Build history of the part. All positions in model axes, mm. A direction names the side the tool comes from. Coordinates: 2 decimals unless noted, no trailing zeros. Write each loop counter-clockwise with the first axis right and the second up, starting at its lowest first coordinate (ties: lowest second). Pieces come first, ordered by that corner, then holes. Notation, with made-up numbers: M -13,12 L 13,12 A26 ccw 13,38 Z; hole C -15,75 d4. An arc over 180 degrees is marked long. Use CSV: the item, a comma, the result in double quotes. Start each with the question number.
```python
from build123d import *

# Parameters (mm, degrees)
SKETCH1_R               = 3.75
BOSS_EXTRUDE1_DEPTH     = 5
CUT_EXTRUDE2_DEPTH      = 2
SKETCH4_R               = 3.75
SKETCH4_R_2             = 2.75
BOSS_EXTRUDE2_DEPTH     = 0.5
SKETCH5_W               = 2
SKETCH5_H               = 5
BOSS_EXTRUDE3_DEPTH     = 2
SKETCH5_2_W             = 2
SKETCH5_2_H             = 5
BOSS_EXTRUDE4_DEPTH     = 12
CUT_EXTRUDE3_DEPTH      = 121.241423811
CUT_EXTRUDE3_DEPTH_BACK = 121.241423811
SKETCH6_R               = 0.75
BOSS_EXTRUDE5_DEPTH     = 5


with BuildPart() as part:
    # Sketch1 → Boss-Extrude1 (new body)
    with BuildSketch(Plane.XY):
        with BuildLine():
            Line((120, 5), (120, -5))
            Line((120, -5), (0, -5))
            ThreePointArc((0, -5), (-5, 0), (0, 5))
            Line((0, 5), (120, 5))
        make_face()
        Circle(SKETCH1_R, mode=Mode.SUBTRACT)
    extrude(amount=BOSS_EXTRUDE1_DEPTH)

    # Sketch3 → Cut-Extrude2 (cut)
    with BuildSketch(Plane(origin=(0, 0, 0), x_dir=(-1, 0, 0), z_dir=(0, 0, -1))):
        with BuildLine():
            Line((-16.129718884, 2.749435925), (0, 4.1))
            ThreePointArc((0, 4.1), (4.1, 0), (0, -4.1))
            Line((0, -4.1), (-16.129718884, -2.749435925))
            ThreePointArc((-16.129718884, -2.749435925), (-18.4, 0), (-16.129718884, 2.749435925))
        make_face()
    extrude(amount=-CUT_EXTRUDE2_DEPTH, mode=Mode.SUBTRACT)

    # Sketch4 → Boss-Extrude2 (add)
    with BuildSketch(Plane(origin=(0, 0, 2), x_dir=(-1, 0, 0), z_dir=(0, 0, -1))):
        Circle(SKETCH4_R)
        Circle(SKETCH4_R_2, mode=Mode.SUBTRACT)
    extrude(amount=-BOSS_EXTRUDE2_DEPTH)

    # Sketch5 → Boss-Extrude3 (add)
    with BuildSketch(Plane(origin=(0, 5, 0), x_dir=(1, 0, 0), z_dir=(0, 1, 0))):
        with Locations((104, -2.5)):
            Rectangle(SKETCH5_W, SKETCH5_H)
    extrude(amount=BOSS_EXTRUDE3_DEPTH)

    # Sketch5<2> → Boss-Extrude4 (add)
    with BuildSketch(Plane(origin=(0, 5, 0), x_dir=(1, 0, 0), z_dir=(0, 1, 0))):
        with Locations((104, -2.5)):
            Rectangle(SKETCH5_2_W, SKETCH5_2_H)
    extrude(amount=-BOSS_EXTRUDE4_DEPTH)

    # Sketch6 → Cut-Extrude3 (cut, two sides: drawn at the far end of the back side and taken through both)
    with BuildSketch(Plane(origin=(0, 0, 2), x_dir=(-1, 0, 0), z_dir=(0, 0, -1)).offset(-CUT_EXTRUDE3_DEPTH_BACK)):
        with Locations((-17.55, 0)):
            Circle(SKETCH6_R)
        with BuildLine():
            ThreePointArc((-15.9, 0), (-15.15, -0.75), (-14.4, 0))
            Line((-14.4, 0), (-15.9, 0))
        make_face()
        with BuildLine():
            Line((-15.9, 0), (-14.4, 0))
            ThreePointArc((-14.4, 0), (-15.15, 0.75), (-15.9, 0))
        make_face()
        with BuildLine():
            ThreePointArc((-13.5, 0), (-12.75, -0.75), (-12, 0))
            Line((-12, 0), (-13.5, 0))
        make_face()
        with BuildLine():
            Line((-13.5, 0), (-12, 0))
            ThreePointArc((-12, 0), (-12.75, 0.75), (-13.5, 0))
        make_face()
        with BuildLine():
            ThreePointArc((-11.1, 0), (-10.35, -0.75), (-9.6, 0))
            Line((-9.6, 0), (-11.1, 0))
        make_face()
        with BuildLine():
            Line((-11.1, 0), (-9.6, 0))
            ThreePointArc((-9.6, 0), (-10.35, 0.75), (-11.1, 0))
        make_face()
        with BuildLine():
            ThreePointArc((-8.7, 0), (-7.95, -0.75), (-7.2, 0))
            Line((-7.2, 0), (-8.7, 0))
        make_face()
        with BuildLine():
            Line((-8.7, 0), (-7.2, 0))
            ThreePointArc((-7.2, 0), (-7.95, 0.75), (-8.7, 0))
        make_face()
    extrude(amount=CUT_EXTRUDE3_DEPTH + CUT_EXTRUDE3_DEPTH_BACK, mode=Mode.SUBTRACT)

    # Sketch7 → Boss-Extrude5 (add)
    with BuildSketch(Plane.XY.offset(5)):
        Polygon((120, 5), (127.743232655, 0), (120, -5), align=None)
    extrude(amount=-BOSS_EXTRUDE5_DEPTH)


solid = part.part
```
1. Slice it at B-B (x = 22.5). List the corners of the cut face in (y, z).
2. Drill centre lines: line 1 along Y through (x, z) = (7.95, 4.25); line 2 along Y through (x, z) = (0, 2.3); line 3 along Y through (x, z) = (28.5, 0.85). Where is each one in solid material? Low to high. Write a range as from..to.
3. 3-axis set-ups, long thin cutter, end or side, ignore diameter. For faces 1 (the flat face through (51, 5, 2)), 2 (the flat face through (7, -1, 2)), 3 (the cylindrical face through (-3.746, 0.165, 3.732)), 4 (the flat face through (113, -5, 2)), 5 (the flat face through (52, -5, 2)): which of +Z, -Z, +X, -X, +Y, -Y reach the whole face in a straight line?
4. Flat gauge pins, fed straight in: pin 1 (8 mm diameter, centred on x = -2, y = 1, fed in from +Z); pin 2 (2.5 mm diameter, centred on x = 12.75, y = 0, fed in from -Z); pin 3 (1.5 mm diameter, centred on x = 72, z = 2, fed in from -Y); pin 4 (1 mm diameter, centred on y = 2.5, z = 1.5, fed in from +X). Where does each tip first touch, or does it go through?
5. Pull direction X, two halves, no side cores. Call faces 6 (the flat face through (112, 5, 2)), 7 (the flat face through (123.926, -2.465, 2.535)), 8 (the cylindrical face through (-4.1, 0.1, 1)), 9 (the cylindrical face through (18.4, -0.1, 1)): pulls with the +X half, pulls with the -X half, needs draft (parallel to the pull), parting line crosses it, or undercut.
6. Slice it at A-A (x = 5). List the corners of the cut face in (y, z).
Established:
1,outline,"M -5,0 L 5,0 L 5,5 L -5,5 Z"
2,line 1,"y = -5..-0.75, 0.75..5"
2,line 2,"y = -5..-2.75, 2.75..5"
2,line 3,"y = -5..5"
3,face 1,"+Z, -Z, -X, +Y"
3,face 2,"-Z"
3,face 3,"+Z"
3,face 4,"+Z, -Z, +X, -Y"
3,face 5,"+Z, -Z, -X, -Y"
4,pin 1,"stops at z = 5"
4,pin 2,"stops at z = 2"
4,pin 3,"stops at y = -5"
4,pin 4,"stops at x = 124.65"
5,face 6,"needs draft"
5,face 7,"pulls with the +X half"
5,face 8,"undercut"
5,face 9,"undercut"
6,outline,"M -5,0 L -3.68,0 L -3.68,2 L 3.68,2 L 3.68,0 L 5,0 L 5,5 L -5,5 Z"
